Design review of the part built by this model. Coordinates are the model's own, in mm. Coordinates: 2 decimals unless noted, no trailing zeros. Loops run counter-clockwise (first coordinate to the right, second up) from the corner with the lowest first, then second, coordinate; pieces in that order, holes last. Notation, with made-up numbers: M -7,55 L 9,55 A21 cw 9,67 Z; hole C 44.5,46 d9. An arc over 180 degrees is marked long. Answer as a JSON object with one key per item and string values. Group by question number.
1. Insertion check: pin 1 (7.5 mm diameter, centred on x = 47.74, z = -169.41, fed in from +Y); pin 2 (8 mm diameter, centred on x = 42.5, z = -104.5, fed in from -Y); pin 3 (4 mm diameter, centred on x = 33.5, z = -151.5, fed in from +Y). Each pin has a flat end and moves straight along its axis. Give the tip position at first contact, or say it passes through.
2. Draft analysis for pull direction Z (two halves, no side actions). For faces 1 (the cylindrical face through (46.523, -32.975, -96.624)), 2 (the flat face through (54.089, -31, -111)), 3 (the cylindrical face through (33.823, -32.975, -96.624)), 4 (the flat face through (41, -25, -48.757)), state which applies: +Z half, -Z half, draft (parallel to the pull), parting line (faces both ways), or undercut.
3. Consider section D-D (z = -138). State the section outline as (x, y) points, then the cut area to 3 significant figures.
4. Consider section C-C (x = 43.25). State the section outline as (y, z) points.
5. Consider section B-B (y = -26.5). State the section outline as (x, z) points (3 decimals), then the cut area to 3 significant figures.
6. To check wall thickness, follow probe 1 along Y at (x, z) = (31.25, -121.5); probe 2 along Y at (x, z) = (47.5, -165.5). State the ranges of each line that lie inside material, in increasing order.
from build123d import *

# Parameters (mm, degrees)
BOSS_EXTRUDE4_DEPTH = 304.8
SKETCH4_OUTSIDE_W   = 384.928
SKETCH4_OUTSIDE_H   = 321.428
SKETCH4_OUTSIDE_W_2 = 25.4
SKETCH4_OUTSIDE_H_2 = 127
CUT_EXTRUDE2_DEPTH  = 150
SKETCH6_R           = 3.175
CUT_EXTRUDE4_DEPTH  = 150
SKETCH5_R           = 3.175
CUT_EXTRUDE5_DEPTH  = 150


with BuildPart() as part:
    # Sketch3 → Boss-Extrude4 (new body)
    with BuildSketch(Plane(origin=(0, 0, 0), x_dir=(0, 0, -1), z_dir=(1, 0, 0))):
        with BuildLine():
            ThreePointArc((232.90669496, 1.961354585), (112.25669496, -30.366715482), (-8.39330504, 1.961354585))
            Line((-8.39330504, 1.961354585), (-8.39330504, -4.052041589))
            ThreePointArc((-8.39330504, -4.052041589), (112.25669496, -36.380111656), (232.90669496, -4.052041589))
            Line((232.90669496, -4.052041589), (232.90669496, 1.961354585))
        make_face()
    extrude(amount=BOSS_EXTRUDE4_DEPTH)

    # Sketch4 outside → Cut-Extrude2 (cut)
    with BuildSketch(Plane(origin=(0, 1.961354585, 0), x_dir=(1, 0, 0), z_dir=(0, 1, 0))):
        with Locations((152.4, 112.257)):
            Rectangle(SKETCH4_OUTSIDE_W, SKETCH4_OUTSIDE_H)
        with Locations((41.389045768, 112.25669496)):
            Rectangle(SKETCH4_OUTSIDE_W_2, SKETCH4_OUTSIDE_H_2, mode=Mode.SUBTRACT)
    extrude(amount=-CUT_EXTRUDE2_DEPTH, mode=Mode.SUBTRACT)

    # Sketch6 → Cut-Extrude4 (cut)
    with BuildSketch(Plane(origin=(0, 1.961354585, 0), x_dir=(1, 0, 0), z_dir=(0, 1, 0))):
        with Locations(Location((35.039045768, 124.95669496, 0), (0, 0, 270))):
            Circle(SKETCH6_R)
        with Locations(Location((47.739045768, 124.95669496, 0), (0, 0, 270))):
            Circle(SKETCH6_R)
        with Locations(Location((35.039045768, 99.55669496, 0), (0, 0, 270))):
            Circle(SKETCH6_R)
        with Locations(Location((47.739045768, 99.55669496, 0), (0, 0, 270))):
            Circle(SKETCH6_R)
    extrude(amount=-CUT_EXTRUDE4_DEPTH, mode=Mode.SUBTRACT)

    # Sketch5 → Cut-Extrude5 (cut)
    with BuildSketch(Plane(origin=(0, 1.961354585, 0), x_dir=(1, 0, 0), z_dir=(0, 1, 0))):
        with Locations(Location((47.739045768, 169.40669496, 0), (0, 0, 270))):
            Circle(SKETCH5_R)
        with Locations(Location((35.039045768, 169.40669496, 0), (0, 0, 270))):
            Circle(SKETCH5_R)
        with Locations(Location((35.039045768, 55.10669496, 0), (0, 0, 270))):
            Circle(SKETCH5_R)
        with Locations(Location((47.739045768, 55.10669496, 0), (0, 0, 270))):
            Circle(SKETCH5_R)
    extrude(amount=-CUT_EXTRUDE5_DEPTH, mode=Mode.SUBTRACT)


solid = part.part
Findings below:
{
 "1": {"pin 1": "stops at y = -22.55", "pin 2": "stops at y = -36.35", "pin 3": "stops at y = -26.82"},
 "2": {"face 1": "undercut", "face 2": "draft", "face 3": "undercut", "face 4": "+Z half"},
 "3": {"outline": "M 28.69,-35 L 54.09,-35 L 54.09,-28.99 L 28.69,-28.99 Z", "area": "153 mm^2"},
 "4": {"outline": "M -27.87,-175.76 L -21.86,-175.76 A241.3 cw -21.86,-48.76 L -27.87,-48.76 A241.3 ccw Z"},
 "5": {"outline": "M 28.689,-175.757 L 54.089,-175.757 L 54.089,-155.281 L 28.689,-155.281 Z; M 28.689,-69.232 L 54.089,-69.232 L 54.089,-48.757 L 28.689,-48.757 Z; hole C 35.039,-169.407 d6.35; hole C 35.039,-55.107 d6.35; hole C 47.739,-169.407 d6.35; hole C 47.739,-55.107 d6.35", "area": "913 mm^2"},
 "6": {"probe 1": "y = -36.2 to -30.19", "probe 2": "y = -30.43 to -24.42"}
}
